```python
from build123d import *

# Parameters (mm, degrees)
EXTRUDE_1_DEPTH     = 12
CUT_EXTRUDE_START   = -5
CUT_EXTRUDE_1_DEPTH = 5
FILLET_1_R          = 3
SKETCH_3_R          = 2.500000000000002
CUT_EXTRUDE_2_DEPTH = 53.009614555387756
SKETCH_4_R          = 1.5
CUT_EXTRUDE_3_DEPTH = 53.009614555387756
FILLET_2_R          = 10


with BuildPart() as part:
    # 草图1 → 拉伸1 (new body)
    with BuildSketch(Plane.XY):
        with BuildLine():
            Line((26.000000000000004, 0), (40.00000000000001, 0))
            Line((40.00000000000001, 0), (40.000000000000014, -27))
            Line((40.000000000000014, -27), (15.231546211727823, -26.99999999999999))
            ThreePointArc((15.231546211727823, -26.99999999999999), (8.78e-15, -31), (-15.231546211727816, -27))
            Line((-15.231546211727816, -27), (-39.999999999999986, -27))
            Line((-39.999999999999986, -27), (-39.99999999999999, 0))
            Line((-39.99999999999999, 0), (-26.000000000000004, 0))
            ThreePointArc((-26.000000000000004, 0), (-4.78e-15, -26.000000000000004), (26.000000000000004, 0))
        make_face()
    extrude(amount=EXTRUDE_1_DEPTH)

    # 草图2 → 切除-拉伸1 (cut)
    with BuildSketch(Plane.XY.offset(12).offset(CUT_EXTRUDE_START)):
        with BuildLine():
            Line((-39.999999999999986, -27), (-15.231546211727814, -26.999999999999996))
            ThreePointArc((-15.231546211727814, -26.999999999999996), (-26.769179409944208, -15.633650684284165), (-30.999999999999993, 0))
            Line((-30.999999999999993, 0), (-39.99999999999999, 0))
            Line((-39.99999999999999, 0), (-39.999999999999986, -27))
        make_face()
        with BuildLine():
            Line((40.00000000000001, 0), (30.999999999999993, 0))
            ThreePointArc((30.999999999999993, 0), (26.769179409944208, -15.633650684284161), (15.231546211727823, -26.99999999999999))
            Line((15.231546211727823, -26.99999999999999), (40.000000000000014, -27))
            Line((40.000000000000014, -27), (40.00000000000001, 0))
        make_face()
    extrude(amount=CUT_EXTRUDE_1_DEPTH, mode=Mode.SUBTRACT)

    # 镜向1: part across plane


with BuildPart() as part_1:
    add(part.part)
    add(part.part.mirror(Plane.XY))

    # 圆角1
    fillet_1_edges = [part_1.edges().sort_by_distance(p)[0] for p in [
        (3.232e-14, -30.99999999999998, 12),
        (-39.999999999999986, -13.5, 7),
        (40.000000000000014, -13.5, 7),
        (40.000000000000014, -13.5, -7),
        (-39.999999999999986, -13.5, -7),
        (3.232e-14, -30.99999999999998, -12),
    ]]
    fillet(fillet_1_edges, radius=FILLET_1_R)

    # 草图3 → 切除-拉伸2 (cut, through all)
    with BuildSketch(Plane(origin=(0, 0, 0), x_dir=(1, 0, 0), z_dir=(0, 1, 0))):
        with Locations(Location((-33.99999999999999, 0, 0), (0, 0, 270))):
            Circle(SKETCH_3_R)
    cut_extrude_2 = extrude(amount=-CUT_EXTRUDE_2_DEPTH, mode=Mode.SUBTRACT)

    # 镜向2: 切除-拉伸2 across plane
    add(cut_extrude_2.mirror(Plane(origin=(0, 0, 0), x_dir=(0, 0, 1), z_dir=(1, 0, 0))), mode=Mode.SUBTRACT)

    # 草图4 → 切除-拉伸3 (cut, through all)
    with BuildSketch(Plane(origin=(0, 0, 0), x_dir=(1, 0, 0), z_dir=(0, 1, 0))):
        with Locations(Location((0, 0, 0), (0, 0, 270))):
            Circle(SKETCH_4_R)
    extrude(amount=-CUT_EXTRUDE_3_DEPTH, mode=Mode.SUBTRACT)

    # 圆角2
    fillet_2_edges = [part_1.edges().sort_by_distance(p)[0] for p in [
        (-15.231546211727814, -26.999999999999996, 0),
        (15.23154621172782, -26.999999999999986, 0),
    ]]
    fillet(fillet_2_edges, radius=FILLET_2_R)


solid = part_1.part
```
Design review of the part built by this model. Coordinates are the model's own, in mm. A direction names the side the tool comes from. Coordinates: 2 decimals unless noted, no trailing zeros. Loops run counter-clockwise (first coordinate to the right, second up) from the corner with the lowest first, then second, coordinate; pieces in that order, holes last.
Q1. Tool access review of faces 5 (the face through (39.1, -13.31, 6.14)), 6 (the face through (29, -27, 0)), 7 (the face through (-29, -27, 0)): name each direction out of +Z, -Z, +X, -X, +Y, -Y from which nothing blocks a thin tool from reaching the whole face with its end or side.
Reported:
face 5: +Z, +X, +Y, -Y
face 6: +Z, -Z, +X, -Y
face 7: +Z, -Z, -X, -Y
Q2. For pin 1 (2 mm diameter, centred on y = -17.5, z = -8.5, fed in from -X); pin 2 (11 mm diameter, centred on x = 30, z = -3, fed in from -Y); pin 3 (4 mm diameter, centred on x = 21.5, z = -9.5, fed in from -Y); pin 4 (12 mm diameter, centred on x = -22, y = -11, fed in from -Z), all flat-tipped, find the tip position at first contact; note any pin that passes through.
Reported:
pin 1: stops at x = -26.24
pin 2: stops at y = -27
pin 3: stops at y = -24.07
pin 4: stops at z = -12
Q3. We need section A-A on x = -34. State the section outline as (y, z) points, and give its area (3 significant figures).
Reported:
outline: (-27, -7) - (0, -7) - (0, -2.5) - (-27, -2.5) - close; (-27, 2.5) - (0, 2.5) - (0, 7) - (-27, 7) - close
area: 243 mm2
Q4. We need section C-C on y = -8.5. State how many separate pieces and enclosed holes the cut face has, and give its area (3 significant figures).
Reported:
separate pieces: 2
enclosed holes: 2
area: 482 mm2
Q5. We need section B-B on z = 0. State the section outline as (x, y) points, and give its area (3 significant figures).
Reported:
outline: (-40, -27) - (-36.5, -27) - (-36.5, 0) - (-40, 0) - close; (-31.5, -27) - (-17.66, -27) arc R10 cw to (-13.36, -27.98) arc R31 ccw to (-1.5, -30.96) - (-1.5, -25.96) arc R26 cw to (-26, 0) - (-31.5, 0) - close; (1.5, -30.96) arc R31 ccw to (13.36, -27.98) arc R10 cw to (17.66, -27) - (31.5, -27) - (31.5, 0) - (26, 0) arc R26 cw to (1.5, -25.96) - close; (36.5, -27) - (40, -27) - (40, 0) - (36.5, 0) - close
area: 896 mm2
Q6. To check wall thickness, follow line 1 (Z direction, x = 34, y = -6); line 2 (X direction, y = -2, z = 1.5); line 3 (X direction, y = -18, z = 0). State the ranges of each line that lie inside material, in increasing order.
Reported:
line 1: z = -7 to -2.5, 2.5 to 7
line 2: x = -40 to -36, -32 to -25.92, 25.92 to 32, 36 to 40
line 3: x = -40 to -36.5, -31.5 to -18.76, 18.76 to 31.5, 36.5 to 40
Q7. The part is to be moulded in two halves that separate along X. For faces 1 (the face through (31.52, -13.31, -0.33)), 2 (the face through (-31.52, -13.31, -0.33)), 3 (the face through (-31, -17, -7)), 4 (the face through (-39.14, -13.69, 6.1)), say which applies: +X half, -X half, draft (parallel to the pull), parting line (faces both ways), or undercut.
Reported:
face 1: undercut
face 2: undercut
face 3: draft
face 4: -X half
